Can you work these out from the drawing? Everything is in mm from the part's minimum corner. A direction names the side the tool comes from. Coordinates: 2 decimals unless noted, no trailing zeros. Loops run counter-clockwise (first coordinate to the right, second up) from the corner with the lowest first, then second, coordinate; pieces in that order, holes last.
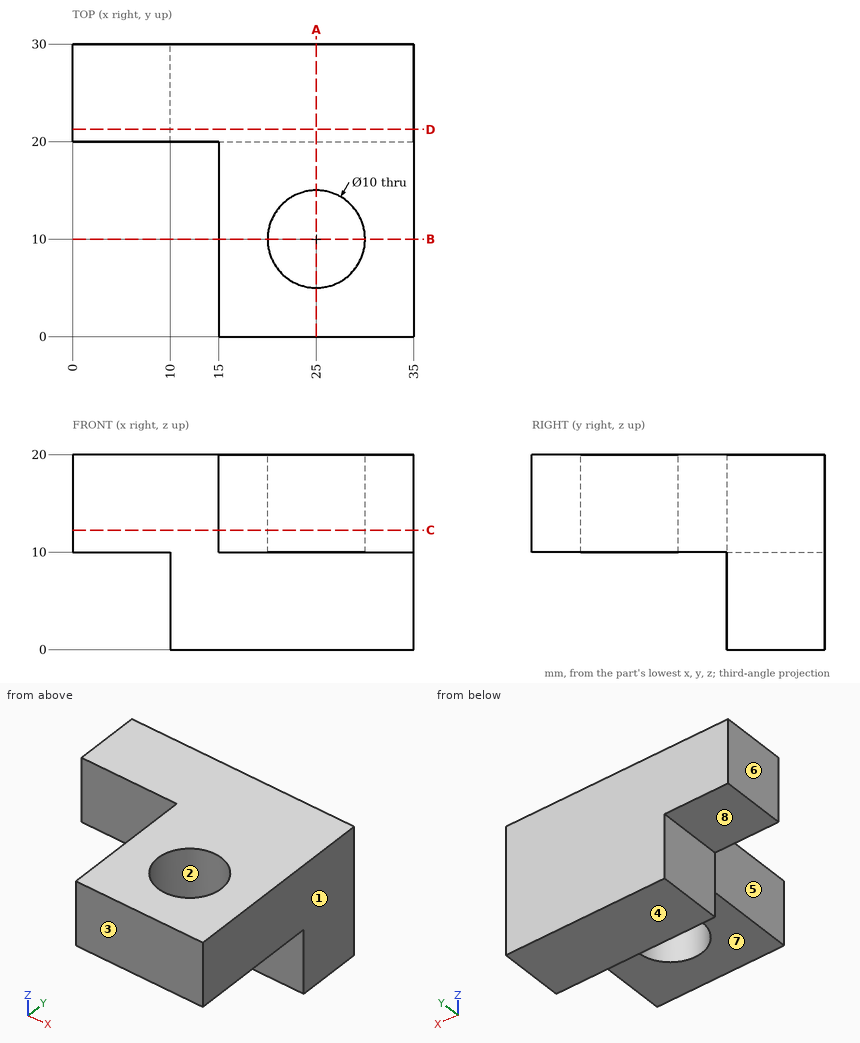
1. I want a section at C-C (z = 12.25). Please give me the cut outline in (x, y).
2. I want a section at A-A (x = 25). Please give me the cut outline in (y, z).
3. On a 3-axis mill with a long thin cutter (end or side, diameter ignored), from which of +Z, -Z, +X, -X, +Y, -Y can I reach the whole of each face in a straight line? I mean the marked faces 4, 5, 6, 7 and 8. Say none if no direction works.
4. I want a section at D-D (y = 21.25). Please give me the cut outline in (x, z), then the cut area to 3 significant figures.
5. I need wall thicknesses on line 1 along Y through (x, z) = (25, 15.25); line 2 along X through (y, z) = (17.25, 11.75); line 3 along Y through (x, z) = (11.5, 3.25). Which ranges of each line are inside material? Lowest first, please.
6. We'd pull the mould along Y, two halves only. Please class the marked faces 1, 2 and 3: +Y half, -Y half, draft (parallel to the pull), parting line (faces both ways), or undercut.
7. For pin 1 (8 mm diameter, centred on y = 9.5, z = 14, fed in from -X); pin 2 (5 mm diameter, centred on x = 17, z = 3, fed in from -Y); pin 3 (3 mm diameter, centred on y = 27, z = 5.5, fed in from -X), each with a flat end and sliding along its axis, tell me the tip position at first contact or that it passes through.
8. I want a section at B-B (y = 10). Please give me the cut outline in (x, z), then the cut area to 3 significant figures.
Response values:
1. outline: (0, 20) - (15, 20) - (15, 0) - (35, 0) - (35, 30) - (0, 30) - close; hole circle Ø10 at (25, 10)
2. outline: (0, 10) - (5, 10) - (5, 20) - (0, 20) - close; (15, 10) - (20, 10) - (20, 0) - (30, 0) - (30, 20) - (15, 20) - close
3. face 4: -Z, +X, -X, +Y, -Y
3. face 5: +Z, -Z, -X, -Y
3. face 6: +Z, -Z, -X, +Y, -Y
3. face 7: -Z, +X, -X, -Y
3. face 8: -Z, -X, +Y, -Y
4. outline: (0, 10) - (10, 10) - (10, 0) - (35, 0) - (35, 20) - (0, 20) - close
4. area: 600 mm2
5. line 1: y = 0 to 5, 15 to 30
5. line 2: x = 15 to 35
5. line 3: y = 20 to 30
6. face 1: draft
6. face 2: undercut
6. face 3: -Y half
7. pin 1: stops at x = 15
7. pin 2: stops at y = 20
7. pin 3: stops at x = 10
8. outline: (15, 10) - (20, 10) - (20, 20) - (15, 20) - close; (30, 10) - (35, 10) - (35, 20) - (30, 20) - close
8. area: 100 mm2
